Build history of the part. All positions in model axes, mm. Face numbers are marked on the shaded views. A direction names the side the tool comes from. Give positions to 0.01 mm unless a question says otherwise; leave off trailing zeros. Loops run counter-clockwise (first coordinate to the right, second up) from the corner with the lowest first, then second, coordinate; pieces in that order, holes last. Notation, with made-up numbers: (56, 21.25) - (90, 21.25) arc R7 cw to (90, 34.25) - close; hole circle Ø5 at (45.25, 25). An arc over 180 degrees is marked (long way). Return JSON: item names as keys, results as strings. Group by question number.
1) 3-axis set-ups, long thin cutter, end or side, ignore diameter. For the marked faces 1, 2, 3 and 4: which of +Z, -Z, +X, -X, +Y, -Y reach the whole face in a straight line?
2) Drop flat-ended pins along their axis: pin 1 (1.5 mm diameter, centred on x = 1.5, y = -5.5, fed in from -Z); pin 2 (6 mm diameter, centred on x = -1.5, z = -3.5, fed in from -Y); pin 3 (8 mm diameter, centred on x = 6.5, z = 3.5, fed in from +Y). Give the stop position or say it passes through.
3) Slice it at B-B (z = -6.5). List the corners of the cut face in (x, y), and give its area (3 significant figures).
4) Slice it at A-A (x = 10). List the corners of the cut face in (y, z).
5) Slice it at C-C (y = -8). List the corners of the cut face in (x, z), and give its area (3 significant figures).
6) Drill centre lines: probe 1 along X at (y, z) = (4.75, -2); probe 2 along X at (y, z) = (-5, 3.4); probe 3 along Y at (x, z) = (10, 1.55). Where is each one in solid material? Low to high. Write a range as from..to.
7) Mould opens along X. For the marked faces 5, 6 and 7 say: released by +X, released by -X, zero draft, split by the parting line, or undercut.
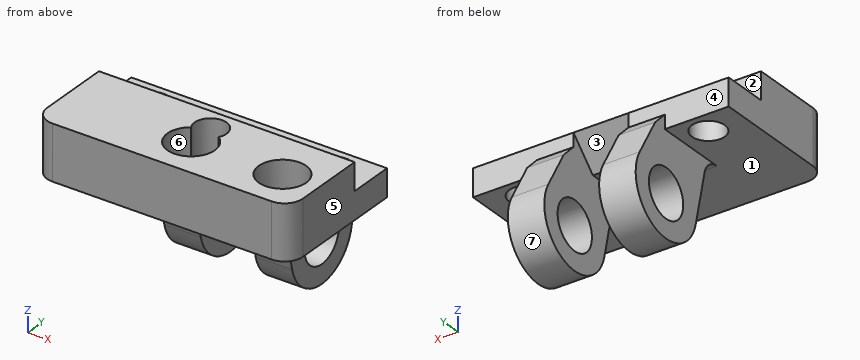
```python
from build123d import *

# Parameters (mm, degrees)
SKETCH1_W           = 28
SKETCH1_H           = 5
BOSS_EXTRUDE1_DEPTH = 3
SKETCH1_3_W         = 28
SKETCH1_3_H         = 10
BOSS_EXTRUDE2_DEPTH = 6
SKETCH2_R           = 1.8
CUT_EXTRUDE1_DEPTH  = 20.006577809
SKETCH3_R           = 2.6
CUT_EXTRUDE2_DEPTH  = 20.704060495
SKETCH4_R           = 1.75
CUT_EXTRUDE3_DEPTH  = 20.704060495
SKETCH5_R           = 2.65
BOSS_EXTRUDE3_DEPTH = 7
SKETCH5_3_R         = 2.65
CUT_EXTRUDE5_DEPTH  = 3
CHAMFER1_SIZE       = 3
CHAMFER2_SIZE       = 1.5
FILLET1_R           = 2


with BuildPart() as part:
    # Sketch1 → Boss-Extrude1 (new body)
    with BuildSketch(Plane.XY):
        Rectangle(SKETCH1_W, SKETCH1_H)
    extrude(amount=BOSS_EXTRUDE1_DEPTH)

    # Sketch1<3> → Boss-Extrude2 (add)
    with BuildSketch(Plane.XY):
        with Locations((0, -7.5)):
            Rectangle(SKETCH1_3_W, SKETCH1_3_H)
    extrude(amount=BOSS_EXTRUDE2_DEPTH)

    # Sketch2 → Cut-Extrude1 (cut, through all)
    with BuildSketch(Plane.XY.offset(3)):
        with Locations((10, 0)):
            Circle(SKETCH2_R)
        with Locations((-10, 0)):
            Circle(SKETCH2_R)
    extrude(amount=-CUT_EXTRUDE1_DEPTH, mode=Mode.SUBTRACT)

    # Sketch3 → Cut-Extrude2 (cut, through all)
    with BuildSketch(Plane.XY.offset(6)):
        with Locations((10, -8)):
            Circle(SKETCH3_R)
        with Locations((0, -8)):
            Circle(SKETCH3_R)
    extrude(amount=-CUT_EXTRUDE2_DEPTH, mode=Mode.SUBTRACT)

    # Sketch4 → Cut-Extrude3 (cut, through all)
    with BuildSketch(Plane(origin=(0, 0, 0), x_dir=(-1, 0, 0), z_dir=(0, 0, -1))):
        with Locations((0, -5)):
            Circle(SKETCH4_R)
    extrude(amount=-CUT_EXTRUDE3_DEPTH, mode=Mode.SUBTRACT)

    # Sketch5 → Boss-Extrude3 (add, symmetric)
    with BuildSketch(Plane(origin=(0, 0, 0), x_dir=(0, 0, -1), z_dir=(1, 0, 0))):
        with BuildLine():
            Line((0, 4), (0, -4))
            Line((0, -4), (7.543277969, -2.282747111))
            ThreePointArc((7.543277969, -2.282747111), (10.879560122, 4.005711915), (4.168926053, 6.381187848))
            Line((4.168926053, 6.381187848), (0, 4))
        make_face()
        with Locations((6.5, 2.3)):
            Circle(SKETCH5_R, mode=Mode.SUBTRACT)
    extrude(amount=BOSS_EXTRUDE3_DEPTH, both=True)

    # Sketch5<3> → Cut-Extrude5 (cut, symmetric)
    with BuildSketch(Plane(origin=(0, 0, 0), x_dir=(0, 0, -1), z_dir=(1, 0, 0))):
        with BuildLine():
            Line((0, 4), (0, -4))
            Line((0, -4), (7.543277969, -2.282747111))
            ThreePointArc((7.543277969, -2.282747111), (10.879560122, 4.005711915), (4.168926053, 6.381187848))
            Line((4.168926053, 6.381187848), (0, 4))
        make_face()
        with Locations((6.5, 2.3)):
            Circle(SKETCH5_3_R, mode=Mode.SUBTRACT)
    extrude(amount=CUT_EXTRUDE5_DEPTH, both=True, mode=Mode.SUBTRACT)

    # Chamfer1
    chamfer1_edges = [part.edges().sort_by_distance(p)[0] for p in [
        (0, 2.5, 0),
    ]]
    chamfer(chamfer1_edges, length=CHAMFER1_SIZE - 0.0001)  # a hair under: the kernel refuses the full size

    # Chamfer2
    chamfer2_edges = [part.edges().sort_by_distance(p)[0] for p in [
        (-5, 2.5, 0),
        (5, 2.5, 0),
    ]]
    chamfer(chamfer2_edges, length=CHAMFER2_SIZE - 0.0001)  # a hair under: the kernel refuses the full size

    # Fillet1
    fillet1_edges = [part.edges().sort_by_distance(p)[0] for p in [
        (-14, -12.5, 3),
        (14, -12.5, 3),
        (5, -4, 0),
        (-5, -4, 0),
    ]]
    fillet(fillet1_edges, radius=FILLET1_R)


solid = part.part
```
Results:
{
 "1": {"face 1": "-Z, -Y", "face 2": "+Z, +X, -X, +Y", "face 3": "-Z, +Y", "face 4": "+Z, +Y"},
 "2": {"pin 1": "z = 0", "pin 2": "y = -3.92", "pin 3": "y = 4.29"},
 "3": {"outline": "(-7, -2.52) - (-3, -2.52) - (-3, -0.35) - (-7, -0.35) - close; (-7, 4.95) - (-3, 4.95) - (-3, 7) - (-7, 7) - close; (3, -2.52) - (7, -2.52) - (7, -0.35) - (3, -0.35) - close; (3, 4.95) - (7, 4.95) - (7, 7) - (3, 7) - close", "area": "33.8 mm2"},
 "4": {"outline": "(-12.5, 0) - (-10.6, 0) - (-10.6, 6) - (-12.5, 6) - close; (-5.4, 0) - (-1.8, 0) - (-1.8, 3) - (-2.5, 3) - (-2.5, 6) - (-5.4, 6) - close; (1.8, 0) - (2.5, 0) - (2.5, 3) - (1.8, 3) - close"},
 "5": {"outline": "(-14, 0) - (-2.6, 0) - (-2.6, 6) - (-14, 6) - close; (2.6, 0) - (7.4, 0) - (7.4, 6) - (2.6, 6) - close; (12.6, 0) - (14, 0) - (14, 6) - (12.6, 6) - close", "area": "106 mm2"},
 "6": {"probe 1": "-7..-3, 3..7", "probe 2": "-14..-1.75, 1.75..14", "probe 3": "-12.5..-10.6, -5.4..-1.8, 1.8..2.5"},
 "7": {"face 5": "released by +X", "face 6": "undercut", "face 7": "zero draft"}
}
